Autodesk Inventor part; units mm, degrees
ref_plane "YZ Plane" through (0, 0, 0) normal (1, 0, 0) x (0, 1, 0)
ref_plane "XZ Plane" through (0, 0, 0) normal (0, 1, 0) x (-1, 0, 0)
ref_plane "XY Plane" through (0, 0, 0) normal (0, 0, 1) x (1, 0, 0)
sketch "Sketch1" plane through (0, 0, 0) normal (0, 0, 1) x (1, 0, 0)
  line L0 (0, 0) -> (485.775, 0)
  line L1 (485.775, 0) -> (485.775, 9.525)
  line L2 (485.775, 9.525) -> (0, 9.525)
  line L3 (0, 9.525) -> (0, 0)
  dimension "d0" = 485.775
  dimension "d1" = 9.525
extrude "Extrusion1" add sketch "Sketch1" along normal blind 187.325
sketch "Sketch2" plane through (0, 0, 187.325) normal (0, 0, 1) x (1, 0, 0)
  line L0 (0, 0) -> (485.775, 0)
  line L1 (485.775, 0) -> (485.775, 9.525)
  line L2 (485.775, 9.525) -> (0, 9.525)
  line L3 (0, 9.525) -> (0, 0)
  line L4 (25.4, 9.525) -> (460.375, 9.525)
  line L5 (460.375, 9.525) -> (460.375, 0)
  line L6 (460.375, 0) -> (25.4, 0)
  line L7 (25.4, 0) -> (25.4, 9.525)
  dimension "d4" = 25.4
  dimension "d5" = 25.4
extrude "Extrusion2" add sketch "Sketch2" along normal blind 9.525 contours L7 L2 L5 L0
mirror "Mirror1" about plane through (242.8875, 4.7625, 0) normal (0, 0, -1)
sketch "Sketch3" plane through (25.4, 9.525, 196.85) normal (0, 1, 0) x (1, 0, 0)
  line L0 (-25.4, 384.175) -> (-25.4, 9.525)
  line L1 (0, 9.525) -> (-25.4, 9.525)
  line L2 (460.375, 384.175) -> (460.375, 9.525)
  line L3 (434.975, 393.7) -> (0, 393.7)
  line L4 (179.3875, 196.85) -> (255.5875, 196.85) construction
  line L5 (179.3875, 165.1) -> (255.5875, 165.1)
  line L6 (255.5875, 228.6) -> (179.3875, 228.6)
  arc A0 (179.3875, 228.6) -> (179.3875, 165.1) centre (179.3875, 196.85) ccw
  arc A1 (255.5875, 165.1) -> (255.5875, 228.6) centre (255.5875, 196.85) ccw
  point P0 (-25.4, 196.85)
  point P1 (217.4875, 196.85)
  dimension "d8" = 76.2
  dimension "d9" = 31.75
  dimension "d10" = 196.85
  dimension "d11" = 242.8875
  dimension "d12" = 242.8875
extrude "Extrusion3" cut sketch "Sketch3" against normal through all
properties part number "top_cover_sheet" material "Wood (Birch)"
Here's how the part is built. I have some questions about the finished solid (model axes, mm). A direction names the side the tool comes from. Give positions to 0.01 mm unless a question says otherwise; leave off trailing zeros. Write each loop counter-clockwise with the first axis right and the second up, starting at its lowest first coordinate (ties: lowest second). Pieces come first, ordered by that corner, then holes.
(1) Will these pins go through, and if not, where does the flat tip stop? pin 1 (3 mm diameter, centred on y = 3.5, z = -193.5, fed in from -X); pin 2 (5 mm diameter, centred on y = 6, z = -192.5, fed in from +X) (3 decimals); pin 3 (5 mm diameter, centred on x = 9.5, y = 6, fed in from +Z) (3 decimals).
Output values:
pin 1: stops at x = 25.4
pin 2: stops at x = 460.375
pin 3: stops at z = 187.325
(2) Imagine slicing it at B-B, the plane x = 257. Write out the boundary of the cut face in (y, z) (3 decimals), and give its area (3 significant figures).
Output values:
outline: (0, -196.85) - (9.525, -196.85) - (9.525, -31.75) - (0, -31.75) - close; (0, 31.75) - (9.525, 31.75) - (9.525, 196.85) - (0, 196.85) - close
area: 3,150 mm2
(3) Imagine slicing it at A-A, the plane z = 0. Write out the boundary of the cut face in (x, y) (1 decimal), and give its area (3 significant figures).
Output values:
outline: (0, 0) - (173, 0) - (173, 9.5) - (0, 9.5) - close; (312.7, 0) - (485.8, 0) - (485.8, 9.5) - (312.7, 9.5) - close
area: 3,300 mm2
(4) Thinking about a two-plate mould opening in X: for faces 1 (the face through (460.375, 5, 192)), 2 (the face through (312.73, 4.83, 0.7)), 3 (the face through (25.4, 5, -192)), 4 (the face through (473, 5, 187.325)), which applies, pulls with the +X half, pulls with the -X half, needs draft (parallel to the pull), parting line crosses it, or undercut?
Output values:
face 1: pulls with the +X half
face 2: undercut
face 3: pulls with the -X half
face 4: needs draft
(5) On a 3-axis mill with a long thin cutter (end or side, diameter ignored), from which of +Z, -Z, +X, -X, +Y, -Y can I reach the whole of each face in a straight line? I mean faces 5 (the face through (240, 5, 196.85)), 6 (the face through (13, 5, -187.325)), 7 (the face through (243, 5, -31.75)), 8 (the face through (473, 5, -187.325)), 9 (the face through (13, 5, 187.325)). Say none if no direction works.
Output values:
face 5: +Z, +X, -X, +Y, -Y
face 6: -Z, -X, +Y, -Y
face 7: +Y, -Y
face 8: -Z, +X, +Y, -Y
face 9: +Z, -X, +Y, -Y
(6) If I drill on L1, parallel to X at y = 5.25, z = 1 (3 decimals); L2, parallel to Z at x = 465, y = 4.5 (3 decimals); L3, parallel to Z at x = 275, y = 6.5, over which ranges is the centre line in solid material (lowest first)?
Output values:
L1: x = 0 to 173.053, 312.722 to 485.775
L2: z = -187.325 to 187.325
L3: z = -196.85 to -31.75, 31.75 to 196.85
